```python
from build123d import *

# Parameters (mm, degrees)
SKETCH1_W           = 218
SKETCH1_H           = 218
SKETCH1_R           = 1.5
SKETCH1_R_2         = 2.65
BOSS_EXTRUDE1_DEPTH = 2
CHAMFER1_SIZE       = 3


with BuildPart() as part:
    # Sketch1 → Boss-Extrude1 (new body)
    with BuildSketch(Plane.XY):
        Rectangle(SKETCH1_W, SKETCH1_H)
        with Locations((-104.526250503, 104.526250503)):
            Circle(SKETCH1_R, mode=Mode.SUBTRACT)
        with Locations((104.473749497, 104.473749497)):
            Circle(SKETCH1_R, mode=Mode.SUBTRACT)
        with Locations((104.526250503, -104.526250503)):
            Circle(SKETCH1_R, mode=Mode.SUBTRACT)
        with Locations((-104.473749497, -104.473749497)):
            Circle(SKETCH1_R, mode=Mode.SUBTRACT)
        with Locations((42.5, 25)):
            Circle(SKETCH1_R_2, mode=Mode.SUBTRACT)
        with Locations((42.5, -25)):
            Circle(SKETCH1_R_2, mode=Mode.SUBTRACT)
        with Locations((-22.5, 99)):
            Circle(SKETCH1_R_2, mode=Mode.SUBTRACT)
        with Locations((22.5, 99)):
            Circle(SKETCH1_R_2, mode=Mode.SUBTRACT)
        with BuildLine():
            Line((-19.85, 56.5), (-19.85, 53.5))
            ThreePointArc((-19.85, 53.5), (-22.5, 50.85), (-25.15, 53.5))
            Line((-25.15, 53.5), (-25.15, 56.5))
            ThreePointArc((-25.15, 56.5), (-22.5, 59.15), (-19.85, 56.5))
        make_face(mode=Mode.SUBTRACT)
        with BuildLine():
            Line((-25.15, 23.5), (-25.15, 26.5))
            ThreePointArc((-25.15, 26.5), (-22.5, 29.15), (-19.85, 26.5))
            Line((-19.85, 26.5), (-19.85, 23.5))
            ThreePointArc((-19.85, 23.5), (-22.5, 20.85), (-25.15, 23.5))
        make_face(mode=Mode.SUBTRACT)
        with BuildLine():
            Line((25.15, 56.5), (25.15, 53.5))
            ThreePointArc((25.15, 53.5), (22.5, 50.85), (19.85, 53.5))
            Line((19.85, 53.5), (19.85, 56.5))
            ThreePointArc((19.85, 56.5), (22.5, 59.15), (25.15, 56.5))
        make_face(mode=Mode.SUBTRACT)
        with BuildLine():
            Line((19.85, 23.5), (19.85, 26.5))
            ThreePointArc((19.85, 26.5), (22.5, 29.15), (25.15, 26.5))
            Line((25.15, 26.5), (25.15, 23.5))
            ThreePointArc((25.15, 23.5), (22.5, 20.85), (19.85, 23.5))
        make_face(mode=Mode.SUBTRACT)
        with BuildLine():
            Line((25.15, -23.5), (25.15, -26.5))
            ThreePointArc((25.15, -26.5), (22.5, -29.15), (19.85, -26.5))
            Line((19.85, -26.5), (19.85, -23.5))
            ThreePointArc((19.85, -23.5), (22.5, -20.85), (25.15, -23.5))
        make_face(mode=Mode.SUBTRACT)
        with BuildLine():
            Line((19.85, -56.5), (19.85, -53.5))
            ThreePointArc((19.85, -53.5), (22.5, -50.85), (25.15, -53.5))
            Line((25.15, -53.5), (25.15, -56.5))
            ThreePointArc((25.15, -56.5), (22.5, -59.15), (19.85, -56.5))
        make_face(mode=Mode.SUBTRACT)
        with BuildLine():
            Line((-19.85, -23.5), (-19.85, -26.5))
            ThreePointArc((-19.85, -26.5), (-22.5, -29.15), (-25.15, -26.5))
            Line((-25.15, -26.5), (-25.15, -23.5))
            ThreePointArc((-25.15, -23.5), (-22.5, -20.85), (-19.85, -23.5))
        make_face(mode=Mode.SUBTRACT)
        with BuildLine():
            Line((-25.15, -56.5), (-25.15, -53.5))
            ThreePointArc((-25.15, -53.5), (-22.5, -50.85), (-19.85, -53.5))
            Line((-19.85, -53.5), (-19.85, -56.5))
            ThreePointArc((-19.85, -56.5), (-22.5, -59.15), (-25.15, -56.5))
        make_face(mode=Mode.SUBTRACT)
    extrude(amount=BOSS_EXTRUDE1_DEPTH)

    # Chamfer1
    chamfer1_edges = [part.edges().sort_by_distance(p)[0] for p in [
        (109, -109, 1),
        (-109, -109, 1),
        (-109, 109, 1),
        (109, 109, 1),
    ]]
    chamfer(chamfer1_edges, length=CHAMFER1_SIZE)


solid = part.part
```
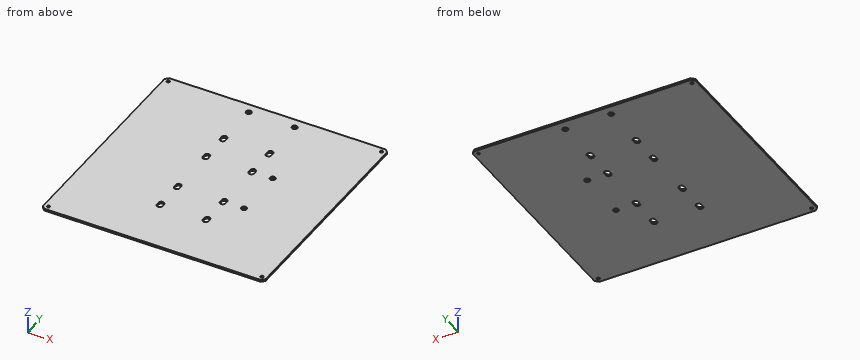
Model file for the job. Use its own axes, mm. Round coordinates to 2 decimals unless told otherwise and drop trailing zeros. Write each loop counter-clockwise with the first axis right and the second up, starting at its lowest first coordinate (ties: lowest second). Pieces come first, ordered by that corner, then holes. Notation, with made-up numbers: (60, 83) - (93, 83) arc R13 ccw to (93, 92) - close; hole circle Ø3 at (-40, 22). An arc over 180 degrees is marked (long way). Use CSV: the item, a comma, the result in double quotes. Start each with the question number.
Item 1: Drill centre lines: L1, parallel to Y at x = 22.5, z = 0.75; L2, parallel to Y at x = 24, z = 0.8; L3, parallel to X at y = -27, z = 1.55. Where is each one in solid material? Low to high. Write a range as [from, to].
Item 2: Pin check, flat tip, straight feed: P1, Ø6, axis at x = 42.5, y = 25, coming from the +Z side. Stop position of the tip, or through.
Item 3: Band-saw the part on A-A (y = 99). Write the cut outline in (x, z), and give its area (3 significant figures).
Item 4: Band-saw the part on B-B (x = 42.5). Write the cut outline in (y, z), and give its area (3 significant figures).
Checked values:
1,L1,"y = [-109, -59.15], [-50.85, -29.15], [-20.85, 20.85], [29.15, 50.85], [59.15, 96.35], [101.65, 109]"
1,L2,"y = [-109, -58.68], [-51.32, -28.68], [-21.32, 21.32], [28.68, 51.32], [58.68, 96.82], [101.18, 109]"
1,L3,"x = [-109, -25.1], [-19.9, 19.9], [25.1, 40.76], [44.24, 109]"
2,P1,"stops at z = 2"
3,outline,"(-109, 0) - (-25.15, 0) - (-25.15, 2) - (-109, 2) - close; (-19.85, 0) - (19.85, 0) - (19.85, 2) - (-19.85, 2) - close; (25.15, 0) - (109, 0) - (109, 2) - (25.15, 2) - close"
3,area,"415 mm²"
4,outline,"(-109, 0) - (-27.65, 0) - (-27.65, 2) - (-109, 2) - close; (-22.35, 0) - (22.35, 0) - (22.35, 2) - (-22.35, 2) - close; (27.65, 0) - (109, 0) - (109, 2) - (27.65, 2) - close"
4,area,"415 mm²"
